```python
from build123d import *

# Parameters (mm, degrees)
F1_DEPTH  = 3.175
F2_R      = 2.3991188234
F3_DEPTH  = 6.35
F5_R      = 4.445
F6_DEPTH  = 25.4
F7_R      = 2.54
F8_R      = 2.54
F9_R      = 2.54
F10_DEPTH = 12.7


with BuildPart() as f1:
    # F0 (on Front) → F1 (new body)
    with BuildSketch(Plane.XZ):
        Polygon((27.2537042447, 5.3584766197), (0, 37.8381765649), (-27.2537042447, 5.3584766197), (-27.2537042447, 0), (27.2537042447, 0), align=None)
    extrude(amount=F1_DEPTH)

    # F2 (on face) → F3 (join)
    with BuildSketch(Plane(origin=(0, 0, 0), x_dir=(-1, 0, 0), z_dir=(0, 1, 0))):
        with Locations((16.764, 3.2841927184)):
            Circle(F2_R)
        with Locations((11.176, 3.1603162362)):
            Circle(F2_R)
        with Locations((5.588, 3.036439754)):
            Circle(F2_R)
        with Locations((22.352, 3.4080692006)):
            Circle(F2_R)
        with Locations((0, 2.9125632718)):
            Circle(F2_R)
        with Locations((-5.5895148385, 2.9125632718)):
            Circle(F2_R)
        with Locations((-11.179029677, 2.9125632718)):
            Circle(F2_R)
        with Locations((-22.358059354, 2.9125632718)):
            Circle(F2_R)
        with Locations((-16.7685445155, 2.9125632718)):
            Circle(F2_R)
    extrude(amount=F3_DEPTH)

    # F5 (on offset) → F6 (join)
    with BuildSketch(Plane.XY.offset(19.05)):
        with Locations((0, -1.302275006)):
            Circle(F5_R)
    extrude(amount=F6_DEPTH)

    # F7
    f7_edges = [f1.edges().sort_by_distance(p)[0] for p in [
        (0, 3.142725, 19.05),
    ]]
    fillet(f7_edges, radius=F7_R)

    # F8
    f8_edges = [f1.edges().sort_by_distance(p)[0] for p in [
        (0, -5.747275, 19.05),
    ]]
    fillet(f8_edges, radius=F8_R)

    # F9 (on face) → F10 (cut)
    with BuildSketch(Plane.XY.offset(44.45)):
        with Locations((0, -1.302275006)):
            Circle(F9_R)
    extrude(amount=-F10_DEPTH, mode=Mode.SUBTRACT)


solid = f1.part
```
Geometry check sheet. Reference: the model listing, model coordinates, mm. A direction names the side the tool comes from. Give positions to 0.01 mm unless a question says otherwise; leave off trailing zeros. Write each loop counter-clockwise with the first axis right and the second up, starting at its lowest first coordinate (ties: lowest second). Pieces come first, ordered by that corner, then holes. Notation, with made-up numbers: (-0.5, 21.5) -> (25.5, 21.5) arc R20 cw to (25.5, 26.5) -> close; hole circle Ø10 at (52, 21). An arc over 180 degrees is marked (long way). One line per question, with ' | ' between items.
Item 1: Depth check by flat-ended pin: pin 1 (4 mm diameter, centred on x = 0, y = -1.5, fed in from -Z); pin 2 (1 mm diameter, centred on x = 14, z = 23.5, fed in from -Y); pin 3 (5 mm diameter, centred on x = 18.5, y = -1, fed in from +Z); pin 4 (6 mm diameter, centred on x = -5, z = 4.5, fed in from -Y) (3 decimals). Enter the tip coordinate at first touch or a pass-through.
Determined:
pin 1: z = 0 | pin 2: through | pin 3: z = 18.77 | pin 4: y = -3.175
Item 2: Sectioned sample at B-B, the plane x = 15.5. Record the boundary of the cut face in (y, z) (3 decimals).
Determined:
outline: (-3.175, 0) -> (0, 0) -> (0, 0.876) -> (6.35, 0.876) -> (6.35, 4.949) -> (0, 4.949) -> (0, 19.366) -> (-3.175, 19.366) -> close
Item 3: Draft check along X on faces 4 (the cylindrical face through (-0.579, 3.105, 32.86)), 5 (the cylindrical face through (17.08, 3.13, 5.29)), 6 (the flat face through (-6, 6.35, 3)). Enter one of: released by +X, released by -X, zero draft, split by the parting line, or undercut.
Determined:
face 4: split by the parting line | face 5: undercut | face 6: zero draft
Item 4: Scan lines: line 1 along Y through (x, z) = (0, 36); line 2 along Y through (x, z) = (13, 19) (3 decimals); line 3 along Z through (x, y) = (0, 6). Record each from-to range of solid material in increasing order.
Determined:
line 1: -5.75 to -3.84, 1.24 to 3.14 | line 2: -3.175 to 0 | line 3: 0.51 to 5.31
Item 5: Sectioned sample at A-A, the plane y = 4. State how many separate pieces and enclosed holes the cut face has, plus the area to 3 significant figures.
Determined:
separate pieces: 9 | enclosed holes: 0 | area: 163 mm^2
Item 6: Sectioned sample at D-D, the plane z = 8.5. Record the boundary of the cut face in (x, y) (3 decimals), plus the area to 3 significant figures.
Determined:
outline: (-24.618, -3.175) -> (24.618, -3.175) -> (24.618, 0) -> (-24.618, 0) -> close | area: 156 mm^2
Item 7: Sectioned sample at C-C, the plane z = 24. Record the boundary of the cut face in (x, y) (3 decimals).
Determined:
outline: (-11.612, -3.175) -> (-4.031, -3.175) arc R4.445 ccw to (4.031, -3.175) -> (11.612, -3.175) -> (11.612, 0) -> (4.25, 0) arc R4.445 ccw to (-4.25, 0) -> (-11.612, 0) -> close
Item 8: Access from +Z, -Z, +X, -X, +Y, -Y to the whole of each face (thin tool, end or side, straight path). Record for faces 1 (the cylindrical face through (-3.19, 3.13, 3.14)), 2 (the flat face through (0, -1, 31.75)), 3 (the flat face through (0, -2, 0)).
Determined:
face 1: +Y | face 2: +Z | face 3: -Z, +X, -X, +Y, -Y
